Input: dimensioned drawing with shaded views. Units: mm. Origin: part minimum x, y, z. A direction names the side the tool comes from. Give positions to 0.01 mm unless a question says otherwise; leave off trailing zeros. Loops run counter-clockwise (first coordinate to the right, second up) from the corner with the lowest first, then second, coordinate; pieces in that order, holes last. Notation, with made-up numbers: (14.25, 22.5) -> (48.25, 22.5) arc R25 cw to (48.25, 51.5) -> close; hole circle Ø2 at (38.5, 40.25). An arc over 180 degrees is marked (long way). Answer in a Markdown table with one row per item. Add a question column.
1) Access query for the marked faces 5 and 6. Directions: +Z, -Z, +X, -X, +Y, -Y. A direction counts if a zero-diameter tool reaches every point of the face in a straight line with its end or side. Return the directions, or none.
2) Draft query along X for the marked faces 1, 2, 3 and 4. Return one class per face: +X half, -X half, draft (parallel to the pull), parting line (faces both ways), or undercut.
3) Section query B-B (z = 45.5). Return the cut outline in (x, y), plus the area to 3 significant figures.
4) Line query: line 1 (X direction, y = 53, z = 37); line 2 (X direction, y = 3, z = 33.5); line 3 (Z direction, x = 41, y = 30.5). Output: solid intervals per line, ascending. Write a range as from..to.
5) Section query D-D (y = 38.5). Return the cut outline in (x, z).
6) Section query A-A (y = 8). Return the cut outline in (x, z).
7) Section query C-C (x = 12.5). Return the cut outline in (y, z).
8) First-contact query: P1, Ø4, axis at x = 58.5, y = 64, coming from the +Z side; P2, Ø11.5, axis at x = 34, y = 49.5, coming from the +Z side; P3, Ø11, axis at x = 7, y = 55.5, coming from the +Z side. Flat tips, straight axial feed; report the tip coordinate or a pass-through.
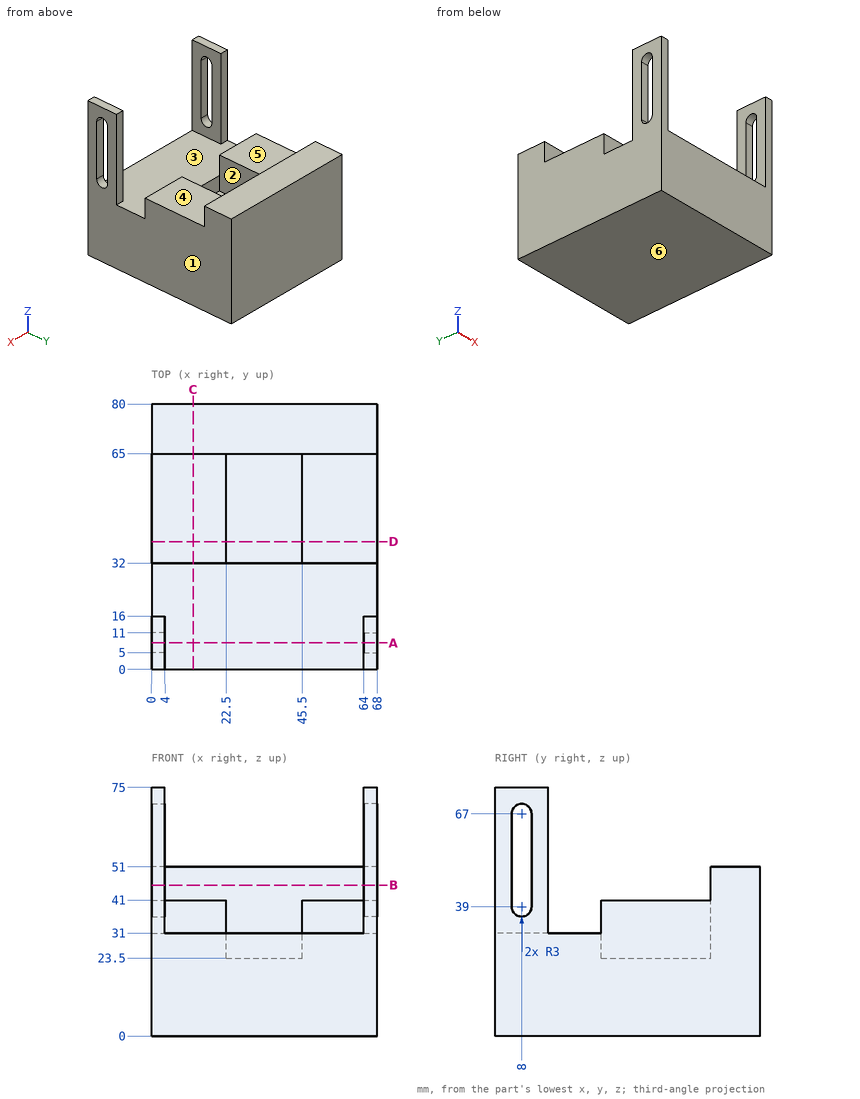
Evaluation:
| question | item | result |
|---|---|---|
| 1 | face 5 | +Z, +X, -X |
| 1 | face 6 | -Z, +X, -X, +Y, -Y |
| 2 | face 1 | +X half |
| 2 | face 2 | undercut |
| 2 | face 3 | undercut |
| 2 | face 4 | draft |
| 3 | outline | (0, 0) -> (4, 0) -> (4, 5) -> (0, 5) -> close; (0, 11) -> (4, 11) -> (4, 16) -> (0, 16) -> close; (0, 65) -> (68, 65) -> (68, 80) -> (0, 80) -> close; (64, 0) -> (68, 0) -> (68, 5) -> (64, 5) -> close; (64, 11) -> (68, 11) -> (68, 16) -> (64, 16) -> close |
| 3 | area | 1,100 mm² |
| 4 | line 1 | 0..22.5, 45.5..68 |
| 4 | line 2 | 0..4, 64..68 |
| 4 | line 3 | 0..31 |
| 5 | outline | (0, 0) -> (68, 0) -> (68, 41) -> (45.5, 41) -> (45.5, 23.5) -> (22.5, 23.5) -> (22.5, 41) -> (0, 41) -> close |
| 6 | outline | (0, 0) -> (68, 0) -> (68, 36) -> (64, 36) -> (64, 31) -> (4, 31) -> (4, 36) -> (0, 36) -> close; (0, 70) -> (4, 70) -> (4, 75) -> (0, 75) -> close; (64, 70) -> (68, 70) -> (68, 75) -> (64, 75) -> close |
| 7 | outline | (0, 0) -> (80, 0) -> (80, 51) -> (65, 51) -> (65, 41) -> (32, 41) -> (32, 31) -> (0, 31) -> close |
| 8 | P1 | z = 51 |
| 8 | P2 | z = 23.5 |
| 8 | P3 | z = 41 |
